```python
from build123d import *

# Parameters (mm, degrees)
SKETCH1_R               = 26
BOSS_EXTRUDE1_DEPTH     = 60
CHAMFER1_SIZE           = 2
CUT_EXTRUDE1_DEPTH      = 116.004347744
CUT_EXTRUDE1_DEPTH_BACK = 116.004347744
SKETCH2_R               = 3


with BuildPart() as part:
    # Sketch1 → Boss-Extrude1 (new body)
    with BuildSketch(Plane.XY):
        with BuildLine():
            Line((-24.387496797, 42.5), (24.387496797, 42.5))
            ThreePointArc((24.387496797, 42.5), (49, 0), (24.387496797, -42.5))
            Line((24.387496797, -42.5), (-24.387496797, -42.5))
            ThreePointArc((-24.387496797, -42.5), (-49, 0), (-24.387496797, 42.5))
        make_face()
        Circle(SKETCH1_R, mode=Mode.SUBTRACT)
    extrude(amount=BOSS_EXTRUDE1_DEPTH)

    # Chamfer1
    chamfer1_edges = [part.edges().sort_by_distance(p)[0] for p in [
        (49, 0, 60),
        (-49, 0, 60),
    ]]
    chamfer(chamfer1_edges, length=CHAMFER1_SIZE)

    # Sketch2 → Cut-Extrude1 (cut, two sides: drawn at the far end of the back side and taken through both)
    with BuildSketch(Plane(origin=(0, 42.5, 0), x_dir=(1, 0, 0), z_dir=(0, 1, 0)).offset(-CUT_EXTRUDE1_DEPTH_BACK)):
        with Locations(Location((0, -30, 0), (0, 0, 180))):
            Circle(SKETCH2_R)
    extrude(amount=CUT_EXTRUDE1_DEPTH + CUT_EXTRUDE1_DEPTH_BACK, mode=Mode.SUBTRACT)


solid = part.part
```
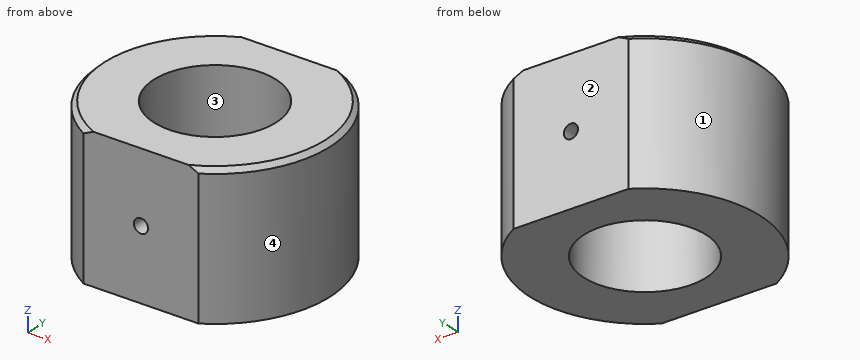
Geometry check sheet. Reference: the model listing, model coordinates, mm. Face numbers are marked on the shaded views. Give positions to 0.01 mm unless a question says otherwise; leave off trailing zeros. Write each loop counter-clockwise with the first axis right and the second up, starting at its lowest first coordinate (ties: lowest second). Pieces come first, ordered by that corner, then holes.
1) Release check for a two-part mould opening along X. For the marked faces 1, 2, 3 and 4 record: pulls with the +X half, pulls with the -X half, needs draft (parallel to the pull), parting line crosses it, or undercut.
2) Gauge pin test, flat ends, axial feed: pin 1 (8 mm diameter, centred on y = 13.5, z = 22, fed in from +X); pin 2 (2 mm diameter, centred on y = -31, z = 14.5, fed in from -X). Record the tip position at first contact, or that the pin passes through.
3) Section check C-C, the plane x = 0. Record the boundary of the cut face in (y, z).
4) Material ranges on L1, parallel to Z at x = 0, y = 35; L2, parallel to X at y = -22, z = 37; L3, parallel to X at y = 33, z = 30, recorded low to high.
5) Section check A-A, the plane y = 0. Record the boundary of the cut face in (x, z), and give its area (3 significant figures).
6) Section check B-B, the plane z = 36. Record the boundary of the cut face in (x, y).
7) Section check D-D, the plane x = -10. Record the boundary of the cut face in (y, z).
Computed:
1. face 1: pulls with the -X half
1. face 2: needs draft
1. face 3: undercut
1. face 4: pulls with the +X half
2. pin 1: stops at x = 48.07
2. pin 2: stops at x = -38.74
3. outline: (-42.5, 0) - (-26, 0) - (-26, 27) - (-42.5, 27) - close; (-42.5, 33) - (-26, 33) - (-26, 60) - (-42.5, 60) - close; (26, 0) - (42.5, 0) - (42.5, 27) - (26, 27) - close; (26, 33) - (42.5, 33) - (42.5, 60) - (26, 60) - close
4. L1: z = 0 to 27, 33 to 60
4. L2: x = -43.78 to -13.86, 13.86 to 43.78
4. L3: x = -36.22 to -3, 3 to 36.22
5. outline: (-49, 0) - (-26, 0) - (-26, 60) - (-47, 60) - (-49, 58) - close; (26, 0) - (49, 0) - (49, 58) - (47, 60) - (26, 60) - close
5. area: 2,760 mm2
6. outline: (-24.39, -42.5) - (24.39, -42.5) arc R49 ccw to (24.39, 42.5) - (-24.39, 42.5) arc R49 ccw to start; hole circle Ø52 at (0, 0)
7. outline: (-42.5, 0) - (-24, 0) - (-24, 60) - (-42.5, 60) - close; (24, 0) - (42.5, 0) - (42.5, 60) - (24, 60) - close
